Check sheet for the modelled part. Datum: model origin and axes. Units: mm. Round coordinates to 2 decimals unless told otherwise and drop trailing zeros. Loops run counter-clockwise (first coordinate to the right, second up) from the corner with the lowest first, then second, coordinate; pieces in that order, holes last. Notation, with made-up numbers: M 38,3.25 L 51,3.25 A35 cw 51,37.25 Z; hole C 33.25,47 d6. An arc over 180 degrees is marked long. One line per question, with ' | ' between items. Start each with the question number.
(1) Thickness scan on probe 1 along Z at (x, y) = (0, 0.1); probe 2 along X at (y, z) = (-5.5, 0). Record the ranges inside material, lowest first. Write a range as [from, to].
(2) Section check D-D (x = -9.25). Record the boundary of the cut face in (y, z), and give its area (3 significant figures).
(3) Section check A-A (x = 0). Record the boundary of the cut face in (y, z), and give its area (3 significant figures).
(4) Go/stop test with flat-tipped pins: P1, Ø3, axis at x = 2.5, z = -1, coming from the -Y side; P2, Ø5, axis at x = 6.5, y = -11.5, coming from the +Z side; P3, Ø1, axis at x = 0, z = 0, coming from the -Y side; P4, Ø3, axis at x = -2.5, y = -13.5, coming from the -Z side. Record where each tip stops, or that it passes through.
(5) Section check C-C (z = -8.75). Record the boundary of the cut face in (x, y), and give its area (3 significant figures).
(6) Section check B-B (z = 0). Record the boundary of the cut face in (x, y).
(7) Draft check along X on faces 1 (the face through (0, 0, -2)), 2 (the face through (11, -17.018, -7)), 3 (the face through (-14.985, -8.505, -0.66)). Enter one of: +X half, -X half, draft (parallel to the pull), parting line (faces both ways), or undercut.
```python
from build123d import *

# Parameters (mm, degrees)
SKETCH1_R           = 15
SKETCH1_R_2         = 0.6
BOSS_EXTRUDE1_DEPTH = 0.25
SKETCH2_R           = 15
SKETCH2_R_2         = 12.815737343
BOSS_EXTRUDE2_DEPTH = 17.268


with BuildPart() as part:
    # Sketch1 → Boss-Extrude1 (new body)
    with BuildSketch(Plane(origin=(0, 0, 0), x_dir=(1, 0, 0), z_dir=(0, 1, 0))):
        Circle(SKETCH1_R)
        Circle(SKETCH1_R_2, mode=Mode.SUBTRACT)
        with BuildLine():
            Line((-12.801684406, 0.6), (-10.235182592, 0.6))
            ThreePointArc((-10.235182592, 0.6), (0, 10.252753907), (10.235182592, 0.6))
            Line((10.235182592, 0.6), (12.801684406, 0.6))
            ThreePointArc((12.801684406, 0.6), (0, 12.815737343), (-12.801684406, 0.6))
        make_face(mode=Mode.SUBTRACT)
        with BuildLine():
            Line((-0.6, 7.600213812), (-0.6, 5.084960781))
            ThreePointArc((-0.6, 5.084960781), (-5.120236922, 0), (-0.6, -5.084960781))
            Line((-0.6, -5.084960781), (-0.6, -7.600213812))
            ThreePointArc((-0.6, -7.600213812), (-7.623860569, 0), (-0.6, 7.600213812))
        make_face(mode=Mode.SUBTRACT)
        with BuildLine():
            Line((0.6, 5.084960781), (0.6, 7.600213812))
            ThreePointArc((0.6, 7.600213812), (7.623860569, 0), (0.6, -7.600213812))
            Line((0.6, -7.600213812), (0.6, -5.084960781))
            ThreePointArc((0.6, -5.084960781), (5.120236922, 0), (0.6, 5.084960781))
        make_face(mode=Mode.SUBTRACT)
        with BuildLine():
            Line((-12.801684406, -0.6), (-10.235182592, -0.6))
            ThreePointArc((-10.235182592, -0.6), (0, -10.252753907), (10.235182592, -0.6))
            Line((10.235182592, -0.6), (12.801684406, -0.6))
            ThreePointArc((12.801684406, -0.6), (0, -12.815737343), (-12.801684406, -0.6))
        make_face(mode=Mode.SUBTRACT)
    extrude(amount=BOSS_EXTRUDE1_DEPTH)

    # Sketch2 → Boss-Extrude2 (add)
    with BuildSketch(Plane(origin=(0, 0.25, 0), x_dir=(1, 0, 0), z_dir=(0, 1, 0))):
        Circle(SKETCH2_R)
        Circle(SKETCH2_R_2, mode=Mode.SUBTRACT)
    extrude(amount=-BOSS_EXTRUDE2_DEPTH)


solid = part.part
```
The answers:
1) probe 1: [-15, -12.82], [-10.25, -0.6], [0.6, 10.25], [12.82, 15] | probe 2: [-15, -12.82], [12.82, 15]
2) outline: M -17.02,-11.81 L 0.25,-11.81 L 0.25,-8.87 L -17.02,-8.87 Z; M -17.02,8.87 L 0.25,8.87 L 0.25,11.81 L -17.02,11.81 Z; M 0,-4.42 L 0.25,-4.42 L 0.25,4.42 L 0,4.42 Z | area: 104 mm²
3) outline: M -17.02,-15 L 0.25,-15 L 0.25,-12.82 L -17.02,-12.82 Z; M -17.02,12.82 L 0.25,12.82 L 0.25,15 L -17.02,15 Z; M 0,-10.25 L 0.25,-10.25 L 0.25,-0.6 L 0,-0.6 Z; M 0,0.6 L 0.25,0.6 L 0.25,10.25 L 0,10.25 Z | area: 80.3 mm²
4) P1: y = 0 | P2: z = 14.46 | P3: through | P4: z = -14.97
5) outline: M -12.18,-17.02 L -9.36,-17.02 L -9.36,0.25 L -12.18,0.25 Z; M -5.34,0 L 5.34,0 L 5.34,0.25 L -5.34,0.25 Z; M 9.36,-17.02 L 12.18,-17.02 L 12.18,0.25 L 9.36,0.25 Z | area: 100 mm²
6) outline: M -15,-17.02 L -12.82,-17.02 L -12.82,0 L -7.62,0 L -7.62,0.25 L -15,0.25 Z; M -5.12,0 L -0.6,0 L -0.6,0.25 L -5.12,0.25 Z; M 0.6,0 L 5.12,0 L 5.12,0.25 L 0.6,0.25 Z; M 7.62,0 L 12.82,0 L 12.82,-17.02 L 15,-17.02 L 15,0.25 L 7.62,0.25 Z
7) face 1: undercut | face 2: draft | face 3: parting line
